Could you check a few things on this model? Use its own coordinates, in mm. A direction names the side the tool comes from. Round coordinates to 2 decimals unless told otherwise and drop trailing zeros. Loops run counter-clockwise (first coordinate to the right, second up) from the corner with the lowest first, then second, coordinate; pieces in that order, holes last.
from build123d import *

# Parameters (mm, degrees)
BOX001_W               = 10
BOX001_H               = 2
BOX001_DEPTH           = 2
BOX001_PLACEMENT_ANGLE = 340
BOX_W                  = 10
BOX_H                  = 2
BOX_DEPTH              = 2
BOX_PLACEMENT_ANGLE    = 40


with BuildPart() as cube001:
    # Box001 → Box001 (new body)
    with BuildSketch(Plane.XY):
        with Locations((5, 1)):
            Rectangle(BOX001_W, BOX001_H)
    extrude(amount=BOX001_DEPTH)


with BuildPart() as cube001_1:
    # Box001 placement: moved
    add(cube001.part.moved(Location((-0.040483, 1.770408, 0))).rotate(Axis((-0.040483, 1.770408, 0), (0, 0, 1)), BOX001_PLACEMENT_ANGLE))


with BuildPart() as fusion:
    # Box → Box (new body)
    with BuildSketch(Plane.XY):
        with Locations((5, 1)):
            Rectangle(BOX_W, BOX_H)
    extrude(amount=BOX_DEPTH)


with BuildPart() as fusion_1:
    # Box placement: moved
    add(fusion.part.moved(Location((2.17, -2.98, 0))).rotate(Axis((2.17, -2.98, 0), (0, 0, 1)), BOX_PLACEMENT_ANGLE))

    # Fusion: union Cube001
    add(cube001_1.part)


solid = fusion_1.part
Item 1: We'd pull the mould along Y, two halves only. Please class faces 6 (the flat face through (8.61, 0.75, 0.99)), 7 (the flat face through (5, 1, 2)), 8 (the flat face through (6.77, 3.49, 0.99)): released by +Y, released by -Y, zero draft, split by the parting line, or undercut.
Results list:
face 6: undercut
face 7: zero draft
face 8: released by +Y
Item 2: If I drill on line 1 along Y through (x, z) = (1, 1.5); line 2 along Y through (x, z) = (8.5, 0.9); line 3 along Y through (x, z) = (6.25, 1.9), over which ranges is the centre line in solid material (lowest first)?
Results list:
line 1: y = -1.59 to -1.35, 1.39 to 3.52
line 2: y = -1.34 to 0.79, 2.33 to 4.94
line 3: y = -0.52 to 3.05
Item 3: If we section it at D-D, the plane y = 4: Please give me the cut outline in (x, z).
Results list:
outline: (7.38, 0) - (9.37, 0) - (9.37, 2) - (7.38, 2) - close
Item 4: If we section it at A-A, the plane y = 2.75: Please give me the cut outline in (x, z), then the cut area to 3 significant figures.
Results list:
outline: (0.32, 0) - (3.12, 0) - (3.12, 2) - (0.32, 2) - close; (5.89, 0) - (9, 0) - (9, 2) - (5.89, 2) - close
area: 11.8 mm2
Item 5: If we section it at B-B, the plane x = 1.75: Please give me the cut outline in (y, z).
Results list:
outline: (-2.48, 0) - (-0.72, 0) - (-0.72, 2) - (-2.48, 2) - close; (1.12, 0) - (3.25, 0) - (3.25, 2) - (1.12, 2) - close
Item 6: If we section it at C-C, the plane z = 1.7: Please give me the cut outline in (x, y).
Results list:
outline: (-0.04, 1.77) - (3.28, 0.56) - (0.88, -1.45) - (2.17, -2.98) - (5.45, -0.23) - (9.36, -1.65) - (10.04, 0.23) - (7.22, 1.26) - (9.83, 3.45) - (8.54, 4.98) - (5.05, 2.05) - (0.64, 3.65) - close
Item 7: For faces 1 (the flat face through (2.065, -0.457, 0.986)), 2 (the flat face through (8.51, 2.34, 0.99)), 3 (the flat face through (2.815, 2.859, 0.986)), 4 (the flat face through (0.297, 2.697, 0.986)), 5 (the flat face through (3.79, -1.62, 0.99)), which set-ups out of +Z, -Z, +X, -X, +Y, -Y let a thin tool reach every point of the face, with its end or its side?
Results list:
face 1: +Z, -Z, -X
face 2: +Z, -Z, +X
face 3: +Z, -Z, +Y
face 4: +Z, -Z, -X, +Y
face 5: +Z, -Z, -Y
